The model under review builds one solid part; all positions refer to its coordinate system, in mm. Face numbers are marked on the shaded views. Give positions to 0.01 mm unless a question says otherwise; leave off trailing zeros. Order: outer loops, then holes, each group sorted by start corner. A loop starts at its lowest first (then second) coordinate and runs counter-clockwise, first axis right, second up. Notation, with made-up numbers: M 67,-28.75 L 114,-28.75 A21 cw 114,-9.75 Z; hole C 77,-14 d7. An arc over 180 degrees is marked long. One line per question, with ' | ' between items. Start each with the question number.
1. Insertion check: P1, Ø3.5, axis at y = -241, z = -15, coming from the +X side; P2, Ø3.5, axis at y = -207.5, z = -15, coming from the -X side. Each pin has a flat end and moves straight along its axis. Give the tip position at first contact, or say it passes through.
2. Wall thickness on L1, parallel to X at y = -346, z = -5; L2, parallel to Z at x = -15.5, y = -343.5; L3, parallel to Y at x = -65.5, z = -14: over which ranges is each line inside the solid? List them lowest first.
3. We need section C-C on y = -247.5. Write out the cut boundary in (x, z), then the cut area to 3 significant figures.
4. The part is to be moulded in two halves that separate along X. For the marked faces 1 and 2, say which applies: +X half, -X half, draft (parallel to the pull), parting line (faces both ways), or undercut.
5. We need section B-B on x = 71.5. Write out the cut boundary in (y, z).
6. We need section D-D on y = -31. Write out the cut boundary in (x, z), then the cut area to 3 significant figures.
7. We need section A-A on z = -4.25. Write out the cut boundary in (x, y).
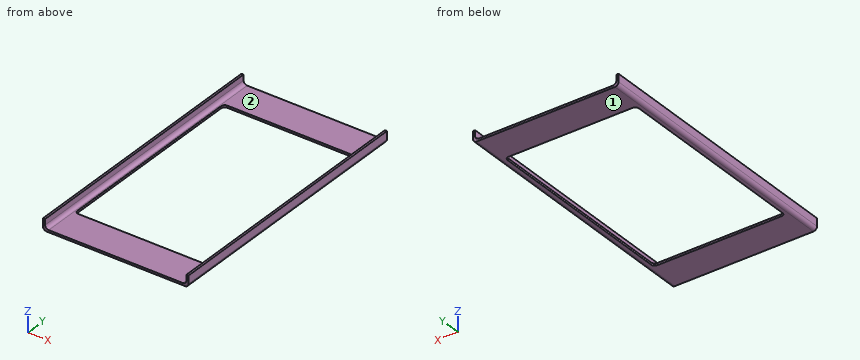
```python
from build123d import *

# Parameters (mm, degrees)
F1_DEPTH = 380
F2_W     = 185
F2_H     = 285
F3_DEPTH = 3
F4_R     = 5
F5_R     = 5
F6_R     = 5


with BuildPart() as f1:
    # F0 (on Front) → F1 (new body)
    with BuildSketch(Plane.XZ):
        Polygon((-102.5, 0), (-102.5, -16), (102.5, -16), (102.5, 0), (99.5, 0), (99.5, -13), (-99.5, -13), (-99.5, 0), align=None)
    extrude(amount=F1_DEPTH)

    # F2 (on face) → F3 (cut)
    with BuildSketch(Plane.XY.offset(-13)):
        with Locations((0, -190)):
            Rectangle(F2_W, F2_H)
    extrude(amount=-F3_DEPTH, mode=Mode.SUBTRACT)

    # F4
    f4_edges = [f1.edges().sort_by_distance(p)[0] for p in [
        (-92.5, -47.5, -14.5),
        (92.5, -47.5, -14.5),
        (-92.5, -332.5, -14.5),
        (92.5, -332.5, -14.5),
    ]]
    fillet(f4_edges, radius=F4_R)

    # F5
    f5_edges = [f1.edges().sort_by_distance(p)[0] for p in [
        (102.5, -190, -16),
        (-102.5, -190, -16),
    ]]
    fillet(f5_edges, radius=F5_R)

    # F6
    f6_edges = [f1.edges().sort_by_distance(p)[0] for p in [
        (-99.5, -190, -13),
        (99.5, -190, -13),
    ]]
    fillet(f6_edges, radius=F6_R)


solid = f1.part
```
Entries:
1) P1: stops at x = 101.97 | P2: stops at x = -101.97
2) L1: x = -102.5 to -99.5, 99.5 to 102.5 | L2: z = -16 to -13 | L3: y = -380 to -332.5, -47.5 to 0
3) outline: M -102.5,-11 A5 ccw -97.5,-16 L -92.5,-16 L -92.5,-13 L -94.5,-13 A5 cw -99.5,-8 L -99.5,0 L -102.5,0 Z; M 92.5,-16 L 97.5,-16 A5 ccw 102.5,-11 L 102.5,0 L 99.5,0 L 99.5,-8 A5 cw 94.5,-13 L 92.5,-13 Z | area: 138 mm^2
4) face 1: draft | face 2: undercut
5) outline: M -380,-16 L -332.5,-16 L -332.5,-13 L -380,-13 Z; M -47.5,-16 L 0,-16 L 0,-13 L -47.5,-13 Z
6) outline: M -102.5,-11 A5 ccw -97.5,-16 L 97.5,-16 A5 ccw 102.5,-11 L 102.5,0 L 99.5,0 L 99.5,-8 A5 cw 94.5,-13 L -94.5,-13 A5 cw -99.5,-8 L -99.5,0 L -102.5,0 Z | area: 693 mm^2
7) outline: M -102.5,-380 L -99.5,-380 L -99.5,0 L -102.5,0 Z; M 99.5,-380 L 102.5,-380 L 102.5,0 L 99.5,0 Z
